Part model, mm, in its own coordinate system. A direction names the side the tool comes from. Give positions to 0.01 mm unless a question says otherwise; leave off trailing zeros. Write each loop counter-clockwise with the first axis right and the second up, starting at its lowest first coordinate (ties: lowest second). Pieces come first, ordered by that corner, then holes.
Autodesk Inventor part; units mm, degrees
ref_plane "YZ Plane" through (0, 0, 0) normal (1, 0, 0) x (0, 1, 0)
ref_plane "XZ Plane" through (0, 0, 0) normal (0, 1, 0) x (-1, 0, 0)
ref_plane "XY Plane" through (0, 0, 0) normal (0, 0, 1) x (1, 0, 0)
sketch "Skizze1" plane through (0, 0, 0) normal (1, 0, 0) x (0, 1, 0)
  line L0 (19.6888, -8.5435) -> (-13.5827, -0.0073)
  arc A0 (-13.5827, -0.0073) -> (-18.2505, -2.2997) centre (-14.5767, -3.8818) ccw
  arc A1 (-18.2505, -2.2997) -> (-23.6613, -28.5435) centre (42.6888, -28.5435) ccw
  line L1 (-23.6613, -28.5435) -> (-23.6613, -91.5435)
  line L2 (-23.6613, -91.5435) -> (19.6888, -91.5435)
  line L3 (19.6888, -91.5435) -> (19.6888, -8.5435)
  circle A2 centre (42.6888, -28.5435) radius 1.621
  arc A3 (-14.3179, -2.9159) -> (-15.3279, -4.5419) centre (-14.5767, -3.8818) ccw
  line L4 (19.6888, -8.5435) -> (19.6888, -44.2151)
  line L5 (-23.6613, -28.5435) -> (42.6888, -28.5435) construction
  dimension "d3" = 83
  dimension "d4" = 3
extrude "Extrusion1" add sketch "Skizze1" along normal blind 35 contours L3 L2 L1 A1 A0 L0
sketch "Skizze2" plane through (35, 0, 0) normal (1, 0, 0) x (0, 0, -1)
  line L0 (8.5435, 19.6888) -> (9.5759, 19.6888)
  line L1 (9.5759, 19.6888) -> (0.976, -13.8312)
  arc A0 (0.976, -13.8312) -> (2.6952, -17.332) centre (3.8818, -14.5767) ccw
  arc A1 (2.6952, -17.332) -> (28.5435, -22.6613) centre (28.5435, 42.6888) ccw
  line L2 (28.5435, -22.6613) -> (91.5435, -22.6613)
  line L3 (91.5435, 19.6888) -> (8.5435, 19.6888)
  line L4 (91.5435, -23.6613) -> (91.5435, 19.6888)
  line L5 (28.5435, -23.6613) -> (91.5435, -23.6613)
  arc A2 (2.2997, -18.2505) -> (28.5435, -23.6613) centre (28.5435, 42.6888) ccw
  arc A3 (0.0073, -13.5827) -> (2.2997, -18.2505) centre (3.8818, -14.5767) ccw
  line L6 (8.5435, 19.6888) -> (0.0073, -13.5827)
  point P0 (0, 0)
extrude "Extrusion2" cut sketch "Skizze2" against normal blind 34 contours L3 L4 L2 A1 A0 L1
sketch "Skizze3" plane through (35, 0, 0) normal (1, 0, 0) x (0, 0, -1)
  line L0 (91.5435, 19.6888) -> (8.5435, 19.6888)
  line L1 (91.5435, -23.6613) -> (91.5435, 19.6888)
  line L2 (28.5435, -23.6613) -> (91.5435, -23.6613)
  arc A0 (2.2997, -18.2505) -> (28.5435, -23.6613) centre (28.5435, 42.6888) ccw
  arc A1 (0.0073, -13.5827) -> (2.2997, -18.2505) centre (3.8818, -14.5767) ccw
  line L3 (8.5435, 19.6888) -> (0.0073, -13.5827)
  point P0 (0, 0)
extrude "Extrusion3" add sketch "Skizze3" along normal blind 1
sketch "Skizze6" plane through (1, 0, 0) normal (1, 0, 0) x (0, 0, -1)
  line L0 (9.5759, 19.6888) -> (91.5435, 19.6888)
  line L1 (9.5759, 19.6888) -> (19.5759, 19.6888)
  line L2 (19.5759, 19.6888) -> (6.1249, 6.2378)
  line L3 (0.976, -13.8312) -> (9.5759, 19.6888)
  point P0 (0, 0)
  dimension "d40" = 10
  dimension "d41" = 45
fillet "Rundung1" radius 2 16 edges at (36, -23.6613, -60.0435) (36, -16.34, -0.2914) (36, 3.0531, -4.2754) (36, -22.2945, -15.1456) (0, -23.6613, -60.0435) (0, -16.34, -0.2914) (0, 3.0531, -4.2754) (0, -22.2945, -15.1456) (1, -21.3151, -15.3475) (1, -15.8991, -1.189) (1, 2.9288, -5.2759) (1, -22.6613, -60.0435) (35, -21.3151, -15.3475) (35, -15.8991, -1.189) (35, 2.9288, -5.2759) (35, -22.6613, -60.0435)
sketch "Skizze4" plane through (0, 19.6888, -10.6083) normal (0, 1, 0) x (1, 0, 0)
  line L0 (0, 80.9352) -> (0, 0)
  line L1 (0, 80.9352) -> (-7, 80.9352)
  line L2 (-7, 80.9352) -> (-7, 65.9352)
  line L3 (-7, 65.9352) -> (0, 65.9352)
  line L4 (0, 65.9352) -> (0, 80.9352)
  circle A0 centre (-3, 72.5285) radius 0.7835
  line L5 (36, 80.9352) -> (36, 0)
  line L6 (36, 80.9352) -> (43, 80.9352)
  line L7 (43, 80.9352) -> (43, 65.9352)
  line L8 (43, 65.9352) -> (36, 65.9352)
  line L9 (36, 65.9352) -> (36, 80.9352)
  circle A1 centre (39, 72.5285) radius 0.7835
  circle A2 centre (-3, 72.5285) radius 1.1
  circle A3 centre (39, 72.5285) radius 1.1
  point P0 (0, -10.6083)
  point P1 (2, 65.9352)
  point P2 (0, -2.0648)
  point P3 (2, -1.0324)
  point P4 (36, 65.9352)
  point P5 (36, 2.9352)
  dimension "d17" = 7
  dimension "d18" = 15
  dimension "d19" = 7
  dimension "d20" = 15
  dimension "d21" = 2.2
  dimension "d22" = 2.2
extrude "Extrusion4" add sketch "Skizze4" against normal blind 2 contours L0 L3 L2 L1 | L6 L7 L8 L5
chamfer "Fasen1" distance 1 angle 45 1 edges at (-4.1, 17.6888, -83.1368)
chamfer "Fasen2" distance 1 angle 45 1 edges at (37.9, 17.6888, -83.1368)
extrude "Extrusion7" add sketch "Skizze6" along normal blind 6
sketch "Skizze8" plane through (35, 0, 0) normal (-1, 0, 0) x (0, 0, 1)
  line L0 (-9.5759, 19.6888) -> (-19.5759, 19.6888)
  line L1 (-91.5435, 19.6888) -> (-8.5435, 19.6888)
  line L2 (-19.5759, 19.6888) -> (-6.1249, 6.2378)
  line L3 (-0.976, -13.8312) -> (-9.5759, 19.6888)
  point P0 (0, 0)
  dimension "d44" = 10
  dimension "d45" = 45
extrude "Extrusion8" add sketch "Skizze8" along normal blind 6
properties part number "verkleidungBremse" material "PC/ABS-Kunststoff, 3DDruck, PLA"
1) Drill centre lines: L1, parallel to X at y = 15.5, z = -14; L2, parallel to X at y = -15.5, z = -69.5; L3, parallel to Z at x = 39, y = 19.4. Where is each one in solid material? Low to high.
Check result:
L1: x = 0 to 7, 29 to 36
L2: x = 0 to 1, 35 to 36
L3: z = -91.54 to -84.24, -82.04 to -76.54
2) Flat gauge pins, fed straight in: P1, Ø3.5, axis at x = -4, z = -83.5, coming from the -Y side; P2, Ø12, axis at y = -8, z = -42, coming from the -X side; P3, Ø8, axis at x = 25.5, z = -31.5, coming from the +Y side. Where does each tip first touch, or does it go through?
Check result:
P1: stops at y = 17.69
P2: stops at x = 0
P3: stops at y = -22.65
3) Saw through at D-D (x = 32). Write the cut outline in (y, z).
Check result:
outline: (-23.66, -91.54) - (-22.66, -91.54) - (-22.66, -28.54) arc R65.35 cw to (-17.33, -2.7) arc R3 cw to (-13.83, -0.98) - (6.24, -6.12) - (19.69, -19.58) - (19.69, -8.54) - (-13.58, -0.01) arc R4 ccw to (-18.25, -2.3) arc R66.35 ccw to (-23.66, -28.54) - close
4) Mould opens along Y. For faces 6 (the flat face through (0, -1, -46)), 7 (the cylindrical face through (35.43, -23.06, -60.48)), 8 (the flat face through (32.042, 13.057, -12.945)), 9 (the cylindrical face through (34.43, -22.06, -60.48)) say: +Y half, -Y half, draft (parallel to the pull), parting line (faces both ways), or undercut.
Check result:
face 6: draft
face 7: -Y half
face 8: undercut
face 9: +Y half
5) 3-axis set-ups, long thin cutter, end or side, ignore diameter. For faces 1 (the flat face through (40, 19, -76.544)), 2 (the flat face through (-1, 19.689, -78)), 3 (the cylindrical face through (18.21, -21.28, -15.17)), 4 (the flat face through (-4, 19, -76.544)), 5 (the cylindrical face through (-2.409, 19.196, -84.064)): which of +Z, -Z, +X, -X, +Y, -Y reach the whole face in a straight line?
Check result:
face 1: +Z, +X, +Y, -Y
face 2: +Z, -Z, +X, -X, +Y
face 3: -Z
face 4: +Z, -X, +Y, -Y
face 5: +Y, -Y
6) Saw through at B-B (x = 24). Write the cut outline in (y, z).
Check result:
outline: (-23.66, -91.54) - (-22.66, -91.54) - (-22.66, -28.54) arc R65.35 cw to (-17.33, -2.7) arc R3 cw to (-13.83, -0.98) - (19.69, -9.58) - (19.69, -8.54) - (-13.58, -0.01) arc R4 ccw to (-18.25, -2.3) arc R66.35 ccw to (-23.66, -28.54) - close
7) Saw through at C-C (z = -38.5). Write the cut outline in (x, y), and give its area (3 significant figures).
Check result:
outline: (0, -21.66) arc R2 ccw to (2, -23.66) - (34, -23.66) arc R2 ccw to (36, -21.66) - (36, 19.69) - (35, 19.69) - (35, -20.66) arc R2 cw to (33, -22.66) - (3, -22.66) arc R2 cw to (1, -20.66) - (1, 19.69) - (0, 19.69) - close
area: 121 mm2
8) Saw through at A-A (x = 39). Write the cut outline in (y, z).
Check result:
outline: (17.69, -91.54) - (19.69, -91.54) - (19.69, -84.24) - (18.69, -84.24) - (17.69, -85.24) - close; (17.69, -81.04) - (18.69, -82.04) - (19.69, -82.04) - (19.69, -76.54) - (17.69, -76.54) - close
